Here's how the part is built. I have some questions about the finished solid (model axes, mm). Face numbers are marked on the shaded views. A direction names the side the tool comes from. Coordinates: 2 decimals unless noted, no trailing zeros. Write each loop counter-clockwise with the first axis right and the second up, starting at its lowest first coordinate (ties: lowest second). Pieces come first, ordered by that corner, then holes.
(1) Thinking about a two-plate mould opening in X: for the marked faces 5, 6, 7 and 8, which applies, released by +X, released by -X, zero draft, split by the parting line, or undercut?
(2) Imagine slicing it at D-D, the plane y = 45. List the corners of the cut face in (x, z) for me.
(3) Imagine slicing it at A-A, the plane y = 7. List the corners of the cut face in (x, z) for me, plus the area to 3 significant figures.
(4) Imagine slicing it at C-C, the plane x = 28. List the corners of the cut face in (y, z) for me.
(5) Which directions (+Z, -Z, +X, -X, +Y, -Y) give clear straight access to the entire face, cutting with the end or side of a thin tool? Please do the marked faces 1, 2, 3 and 4.
(6) Imagine slicing it at B-B, the plane z = 4.25. State how many separate pieces and enclosed holes the cut face has, plus the area to 3 significant figures.
(7) For pin 1 Ø1.1 at (y, z) = (5, 5.5) entering from +X; pin 2 Ø1.6 at (y, z) = (55, 4) entering from -X; pin 3 Ø4 at (x, z) = (18, 2) entering from -Y; pin 4 Ø1.6 at (y, z) = (55, 4.5) entering from +X, each with a flat end and sliding along its axis, tell me the tip position at first contact or that it passes through.
(8) Please list where these lines run through material, in increasing order: probe 1 along X at (y, z) = (51, 3); probe 2 along Y at (x, z) = (49.5, 7); probe 3 along Y at (x, z) = (50.5, 2.75).
Autodesk Fusion 360 part; units mm, degrees
sketch "Sketch1" plane through (0, 0, 0) normal (0, 0, 1) x (1, 0, 0)
  line L0 (0, 0) -> (67, 0)
  line L1 (67, 0) -> (67, 60)
  line L2 (67, 60) -> (0, 60)
  line L3 (0, 60) -> (0, 0)
  dimension "d1" = 67
  dimension "d2" = 60
extrude "Extrude1" add sketch "Sketch1" along normal blind 1 makes body 1
sketch "Sketch2" plane through (0, 0, 1) normal (0, 0, 1) x (-1, 0, 0)
  line L0 (0, -60) -> (0, 0)
  line L1 (0, 0) -> (-67, 0)
  line L2 (-67, 0) -> (-67, -60)
  line L3 (-67, -60) -> (0, -60)
  line L4 (-57, -60) -> (-57, 0)
  line L5 (-10.9779, -55.8771) -> (-7.8284, -57.5781)
  line L6 (-7.8284, -57.5781) -> (-4.7804, -55.701)
  line L7 (-4.7804, -55.701) -> (-4.8821, -52.1229)
  line L8 (-4.8821, -52.1229) -> (-8.0316, -50.4219)
  line L9 (-8.0316, -50.4219) -> (-11.0796, -52.299)
  line L10 (-11.0796, -52.299) -> (-10.9779, -55.8771)
  line L11 (-12.43, -56.5981) -> (-7.93, -59.1962)
  line L12 (-7.93, -59.1962) -> (-3.43, -56.5981)
  line L13 (-3.43, -56.5981) -> (-3.43, -51.4019)
  line L14 (-3.43, -51.4019) -> (-7.93, -48.8038)
  line L15 (-7.93, -48.8038) -> (-12.43, -51.4019)
  line L16 (-12.43, -51.4019) -> (-12.43, -56.5981)
  line L17 (-53.1, -55.7898) -> (-50, -57.5796)
  line L18 (-50, -57.5796) -> (-46.9, -55.7898)
  line L19 (-46.9, -55.7898) -> (-46.9, -52.2102)
  line L20 (-46.9, -52.2102) -> (-50, -50.4204)
  line L21 (-50, -50.4204) -> (-53.1, -52.2102)
  line L22 (-53.1, -52.2102) -> (-53.1, -55.7898)
  line L23 (-54.4959, -56.6052) -> (-49.9918, -59.1961)
  line L24 (-49.9918, -59.1961) -> (-45.4959, -56.5909)
  line L25 (-45.4959, -56.5909) -> (-45.5041, -51.3948)
  line L26 (-45.5041, -51.3948) -> (-50.0082, -48.8039)
  line L27 (-50.0082, -48.8039) -> (-54.5041, -51.4091)
  line L28 (-54.5041, -51.4091) -> (-54.4959, -56.6052)
  line L29 (-11.03, -7.7498) -> (-7.93, -9.5396)
  line L30 (-7.93, -9.5396) -> (-4.83, -7.7498)
  line L31 (-4.83, -7.7498) -> (-4.83, -4.1702)
  line L32 (-4.83, -4.1702) -> (-7.93, -2.3804)
  line L33 (-7.93, -2.3804) -> (-11.03, -4.1702)
  line L34 (-11.03, -4.1702) -> (-11.03, -7.7498)
  line L35 (-12.43, -8.5581) -> (-7.93, -11.1562)
  line L36 (-7.93, -11.1562) -> (-3.43, -8.5581)
  line L37 (-3.43, -8.5581) -> (-3.43, -3.3619)
  line L38 (-3.43, -3.3619) -> (-7.93, -0.7638)
  line L39 (-7.93, -0.7638) -> (-12.43, -3.3619)
  line L40 (-12.43, -3.3619) -> (-12.43, -8.5581)
  line L41 (-52.17, -7.7898) -> (-49.07, -9.5796)
  line L42 (-49.07, -9.5796) -> (-45.97, -7.7898)
  line L43 (-45.97, -7.7898) -> (-45.97, -4.2102)
  line L44 (-45.97, -4.2102) -> (-49.07, -2.4204)
  line L45 (-49.07, -2.4204) -> (-52.17, -4.2102)
  line L46 (-52.17, -4.2102) -> (-52.17, -7.7898)
  line L47 (-53.57, -8.5981) -> (-49.07, -11.1962)
  line L48 (-49.07, -11.1962) -> (-44.57, -8.5981)
  line L49 (-44.57, -8.5981) -> (-44.57, -3.4019)
  line L50 (-44.57, -3.4019) -> (-49.07, -0.8038)
  line L51 (-49.07, -0.8038) -> (-53.57, -3.4019)
  line L52 (-53.57, -3.4019) -> (-53.57, -8.5981)
  point P0 (-7.93, -5.96)
  point P1 (-7.93, -54)
  point P2 (-50, -54)
  point P3 (-49.07, -6)
  point P4 (-7.93, -54)
  point P5 (-7.93, -54)
  point P6 (-50, -54)
  point P7 (-50, -54)
  point P8 (-7.93, -5.96)
  point P9 (-7.93, -5.96)
  point P10 (-49.07, -6)
  point P11 (-49.07, -6)
  dimension "d5" = 48.04
  dimension "d7" = 42.07
  dimension "d8" = 7
  dimension "d9" = 6
  dimension "d10" = 3.1
  dimension "d11" = 4.5
  dimension "d12" = 3.1
  dimension "d13" = 4.5
  dimension "d14" = 3.1
  dimension "d15" = 4.5
  dimension "d16" = 3.1
  dimension "d17" = 4.5
extrude "Extrude2" add sketch "Sketch2" along normal blind 7 contours L11 L12 L13 L14 L15 L16 | L23 L24 L25 L26 L27 L28 | L35 L36 L37 L38 L39 L40 | L47 L48 L49 L50 L51 L52 bodies 1
extrude "Extrude3" cut 1 faces at (67, 20, 0.3333) along direction (-1, 0, 0) blind 9 on bodies 1 bodies 1
extrude "Extrude4" add 4 faces at (8.9799, 53.433, 1) (51.0333, 53.4034, 1) (48.0367, 5.4034, 1) (8.9633, 6.5566, 1) along direction (0, 0, 1) blind 1 on bodies 1 bodies 1
copy_body "Body->Comp1" bodies 1 removing the originals makes body 2 in component "Component"
component "Component" placed x (1, 0, 0) y (0, 1, 0) z (0, 0, 1) at (0, 0, 0)
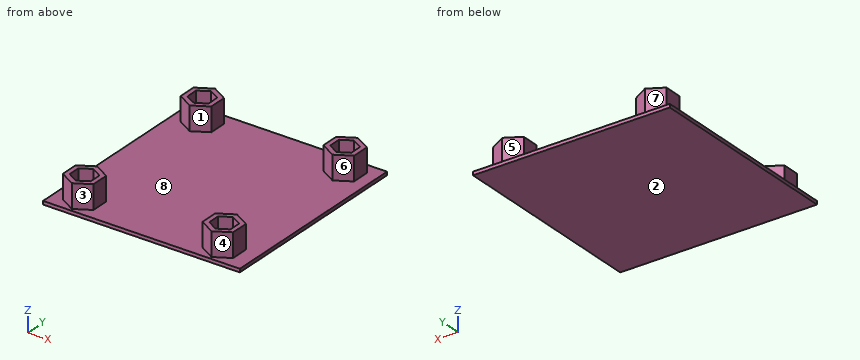
Recorded:
1. face 5: undercut
1. face 6: released by +X
1. face 7: released by -X
1. face 8: undercut
2. outline: (0, 0) - (58, 0) - (58, 1) - (0, 1) - close
3. outline: (0, 0) - (58, 0) - (58, 1) - (53.57, 1) - (53.57, 8) - (52.17, 8) - (52.17, 2) - (45.97, 2) - (45.97, 8) - (44.57, 8) - (44.57, 1) - (12.43, 1) - (12.43, 8) - (11.03, 8) - (11.03, 2) - (4.83, 2) - (4.83, 8) - (3.43, 8) - (3.43, 1) - (0, 1) - close
3. area: 110 mm2
4. outline: (0, 0) - (60, 0) - (60, 1) - (0, 1) - close
5. face 1: +Z
5. face 2: -Z, +X, -X, +Y, -Y
5. face 3: +Z, -Y
5. face 4: +Z, +X, -Y
6. separate pieces: 4
6. enclosed holes: 4
6. area: 147 mm2
7. pin 1: stops at x = 53.57
7. pin 2: stops at x = 3.43
7. pin 3: stops at y = 0
7. pin 4: stops at x = 54.5
8. probe 1: x = 4.13 to 6.96, 8.97 to 11.73, 46.19 to 49, 51 to 53.8
8. probe 2: y = 1.05 to 2.67, 9.33 to 10.95, 49.1 to 50.71, 57.29 to 58.91
8. probe 3: y = 1.63 to 3.25, 8.75 to 10.37, 49.09 to 50.71, 57.29 to 58.9
